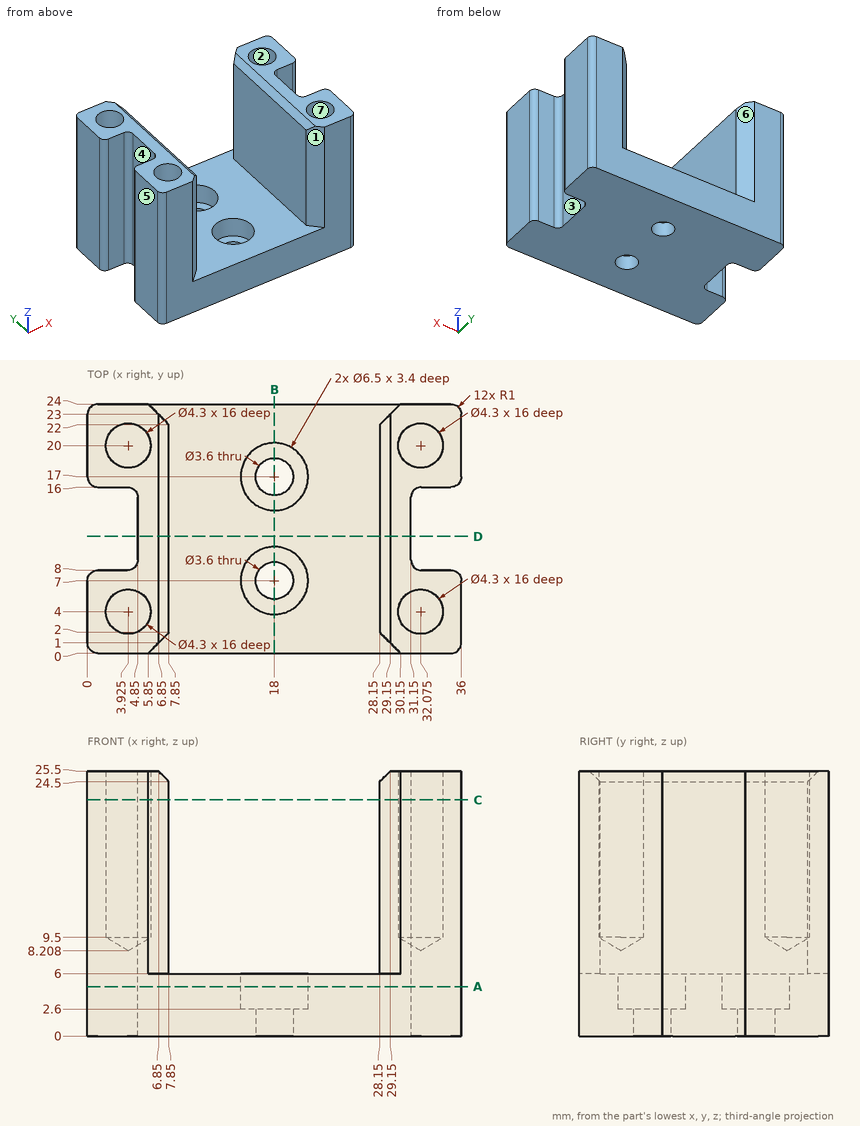
Answer from the drawing. Dimensions are ordinates in mm from the lowest x, y and z of the part. A direction names the side the tool comes from. Give positions to 0.01 mm unless a question says otherwise; leave off trailing zeros. Loops run counter-clockwise (first coordinate to the right, second up) from the corner with the lowest first, then second, coordinate; pieces in that order, holes last.
Item 1: Each of these flat-tipped pins is pushed along its axis until it touches: pin 1 Ø3 at (x, y) = (16.5, 6) entering from +Z; pin 2 Ø5 at (y, z) = (13, 4.5) entering from -X; pin 3 Ø3 at (y, z) = (11.5, 12.5) entering from -X; pin 4 Ø1 at (x, z) = (20, 7.5) entering from -Y. Where does it stop, or does it pass through?
Item 2: The part is cut by section C-C (z = 22.75). Give the number of separate pieces and of enclosed holes in the cut face, and give its area (3 significant figures).
Item 3: The part is cut by section B-B (x = 18). Write down the section's boundary in (y, z).
Item 4: For the marked faces 1, 2, 3 and 4, determine the directions among +Z, -Z, +X, -X, +Y, -Y from which every point of the face is accessible in a straight line to the end or side of a thin tool.
Item 5: Find the intervals of material crossed by line 1 along Y through (x, z) = (18, 0.8); line 2 along X through (y, z) = (20, 17.5) (3 decimals); line 3 along Y through (x, z) = (34, 3), in increasing order.
Item 6: The mould has two halves that part along Y. Classify the marked faces 5, 6 and 7: released by +Y, released by -Y, zero draft, split by the parting line, or undercut.
Item 7: The part is cut by section A-A (z = 4.75). Write down the section's boundary in (x, y), and give its area (3 significant figures).
Item 8: The part is cut by section D-D (y = 11.25). Write down the section's boundary in (x, z).
Taken from the geometry:
1. pin 1: stops at z = 6
1. pin 2: stops at x = 4.72
1. pin 3: stops at x = 4.85
1. pin 4: passes through
2. separate pieces: 2
2. enclosed holes: 4
2. area: 232 mm2
3. outline: (0, 0) - (5.2, 0) - (5.2, 2.6) - (3.75, 2.6) - (3.75, 6) - (0, 6) - close; (8.8, 0) - (15.2, 0) - (15.2, 2.6) - (13.75, 2.6) - (13.75, 6) - (10.25, 6) - (10.25, 2.6) - (8.8, 2.6) - close; (18.8, 0) - (24, 0) - (24, 6) - (20.25, 6) - (20.25, 2.6) - (18.8, 2.6) - close
4. face 1: +Z, -Y
4. face 2: +Z
4. face 3: +Z, -Z, +X
4. face 4: +Z, -Z, -X
5. line 1: y = 0 to 5.2, 8.8 to 15.2, 18.8 to 24
5. line 2: x = 0 to 1.775, 6.075 to 7.85, 28.15 to 29.925, 34.225 to 36
5. line 3: y = 0 to 8, 16 to 24
6. face 5: zero draft
6. face 6: released by +Y
6. face 7: undercut
7. outline: (0, 1) arc R1 ccw to (1, 0) - (35, 0) arc R1 ccw to (36, 1) - (36, 7) arc R1 ccw to (35, 8) - (32.15, 8) arc R1 cw to (31.15, 9) - (31.15, 15) arc R1 cw to (32.15, 16) - (35, 16) arc R1 ccw to (36, 17) - (36, 23) arc R1 ccw to (35, 24) - (1, 24) arc R1 ccw to (0, 23) - (0, 17) arc R1 ccw to (1, 16) - (3.85, 16) arc R1 cw to (4.85, 15) - (4.85, 9) arc R1 cw to (3.85, 8) - (1, 8) arc R1 ccw to (0, 7) - close; hole circle Ø6.5 at (18, 7); hole circle Ø6.5 at (18, 17)
7. area: 719 mm2
8. outline: (4.85, 0) - (31.15, 0) - (31.15, 25.5) - (29.15, 25.5) - (28.15, 24.5) - (28.15, 6) - (7.85, 6) - (7.85, 24.5) - (6.85, 25.5) - (4.85, 25.5) - close
